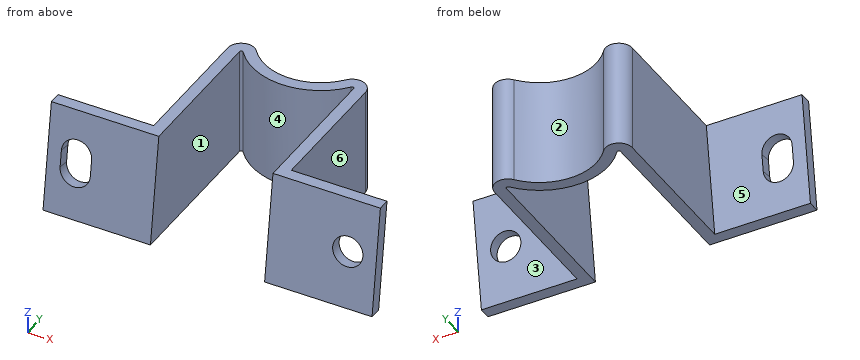
from build123d import *

# Parameters (mm, degrees)
EXTRUDE_1_DEPTH     = 16
CUT_EXTRUDE_1_DEPTH = 50
EXTRUDE_2_DEPTH     = 28.5
SKETCH_4_R          = 4.5
CUT_EXTRUDE_2_DEPTH = 28.5


with BuildPart() as part:
    # 草图1 → 凸台-拉伸1 (new, symmetric)
    with BuildSketch(Plane.XY):
        with BuildLine():
            Line((-17, -12.990381057), (-17, -66.86388681))
            Line((-17, -66.86388681), (-20.5, -66.86388681))
            Line((-20.5, -66.86388681), (-20.5, -12.990381057))
            ThreePointArc((-20.5, -12.990381057), (-17.809307341, -9.210736327), (-13.357142857, -10.51602276))
            ThreePointArc((-13.357142857, -10.51602276), (0, -17), (13.357142857, -10.51602276))
            ThreePointArc((13.357142857, -10.51602276), (17.809307341, -9.210736327), (20.5, -12.990381057))
            Line((20.5, -12.990381057), (20.5, -66.86388681))
            Line((20.5, -66.86388681), (17, -66.86388681))
            Line((17, -66.86388681), (17, -12.990381057))
            ThreePointArc((17, -12.990381057), (16.663663418, -12.517925466), (16.107142857, -12.68108627))
            ThreePointArc((16.107142857, -12.68108627), (0, -20.5), (-16.107142857, -12.68108627))
            ThreePointArc((-16.107142857, -12.68108627), (-16.663663418, -12.517925466), (-17, -12.990381057))
        make_face()
    extrude(amount=EXTRUDE_1_DEPTH, both=True)

    # 草图2 → 切除-拉伸1 (cut, symmetric)
    with BuildSketch(Plane(origin=(0, 0, 0), x_dir=(0, 0, -1), z_dir=(1, 0, 0))):
        Polygon((16, -60.748653355), (-16, -56.251346645), (-16, -66.86388681), (16, -66.86388681), align=None)
    extrude(amount=CUT_EXTRUDE_1_DEPTH, both=True, mode=Mode.SUBTRACT)

    # 草图3 → 凸台-拉伸2 (add)
    with BuildSketch(Plane.ZY.offset(20.5)):
        Polygon((-16, -60.748653355), (16, -56.251346645), (16, -52.716950141), (-16, -57.214256851), align=None)
    extrude_2 = extrude(amount=EXTRUDE_2_DEPTH)

    # 镜向1: 凸台-拉伸2 across plane
    add(extrude_2.mirror(Plane(origin=(0, 0, 0), x_dir=(0, 0, 1), z_dir=(1, 0, 0))))

    # 草图4 → 切除-拉伸2 (cut)
    with BuildSketch(Plane(origin=(0, -53.900966366, 7.575286804), x_dir=(1, 0, 0), z_dir=(0, 0.9902680687415715, -0.13917310096005808))):
        with Locations(Location((40.5, 7.649733485, 0), (0, 0, 270))):
            Circle(SKETCH_4_R)
        with BuildLine():
            Line((-36, 10.149733485), (-36, 5.149733485))
            ThreePointArc((-36, 5.149733485), (-40.5, 0.649733485), (-45, 5.149733485))
            Line((-45, 5.149733485), (-45, 10.149733485))
            ThreePointArc((-45, 10.149733485), (-40.5, 14.649733485), (-36, 10.149733485))
        make_face()
    extrude(amount=-CUT_EXTRUDE_2_DEPTH, mode=Mode.SUBTRACT)


solid = part.part
Read the model definition and answer for the solid it produces. Units are mm, in the model's axes. Face numbers are marked on the shaded views. A direction names the side the tool comes from. Round coordinates to 2 decimals unless told otherwise and drop trailing zeros. Write each loop counter-clockwise with the first axis right and the second up, starting at its lowest first coordinate (ties: lowest second). Pieces come first, ordered by that corner, then holes.
Q1. Find section A-A on y = -36.5. Determine the outline of the cut face in (x, z), and give its area (3 significant figures).
Values:
outline: (-20.5, -16) - (-17, -16) - (-17, 16) - (-20.5, 16) - close; (17, -16) - (20.5, -16) - (20.5, 16) - (17, 16) - close
area: 224 mm2
Q2. Flat-ended cylindrical pins translate along their axes: P1, Ø8, axis at x = -2.5, z = 6, coming from the +Y side; P2, Ø10, axis at y = -30, z = 11.5, coming from the +X side; P3, Ø16, axis at y = -48.5, z = -6.5, coming from the -X side; P4, Ø5, axis at x = -32.5, z = -2, coming from the -Y side. Find the tip coordinate at first contact, or state that the pin passes through.
Values:
P1: stops at y = -15.71
P2: stops at x = 20.5
P3: stops at x = -49
P4: stops at y = -59.13
Q3. Find section C-C on y = -16. Determine the outline of the cut face in (x, z), and give its area (3 significant figures).
Values:
outline: (-20.5, -16) - (-17, -16) - (-17, 16) - (-20.5, 16) - close; (-12.82, -16) - (-5.74, -16) - (-5.74, 16) - (-12.82, 16) - close; (5.74, -16) - (12.82, -16) - (12.82, 16) - (5.74, 16) - close; (17, -16) - (20.5, -16) - (20.5, 16) - (17, 16) - close
area: 677 mm2
Q4. The mould has two halves that part along X. Classify the marked faces 4, 5 and 6: released by +X, released by -X, zero draft, split by the parting line, or undercut.
Values:
face 4: undercut
face 5: zero draft
face 6: released by +X
Q5. Find section D-D on z = -11.5. Determine the outline of the cut face in (x, y), and give its area (3 significant figures).
Values:
outline: (-49, -60.12) - (-17, -60.12) - (-17, -12.99) arc R0.5 cw to (-16.11, -12.68) arc R20.5 ccw to (16.11, -12.68) arc R0.5 cw to (17, -12.99) - (17, -60.12) - (49, -60.12) - (49, -56.58) - (20.5, -56.58) - (20.5, -12.99) arc R4 ccw to (13.36, -10.52) arc R17 cw to (-13.36, -10.52) arc R4 ccw to (-20.5, -12.99) - (-20.5, -56.58) - (-49, -56.58) - close
area: 689 mm2
Q6. A tool of negligible diameter and unlimited length cuts with its end or side. For the marked faces 1, 2 and 3, from which of +Z, -Z, +X, -X, +Y, -Y can it reach the whole face along a straight path? Write none if from no direction.
Values:
face 1: +Z, -Z, -Y
face 2: +Z, -Z, +Y
face 3: -Z, +X, +Y
Q7. Find section B-B on x = -37.5. Determine the outline of the cut face in (y, z), and give its area (3 significant figures).
Values:
outline: (-60.75, -16) - (-57.21, -16) - (-55.78, -5.8) - (-59.25, -5.31) - close; (-57.62, 6.28) - (-54.15, 5.8) - (-52.72, 16) - (-56.25, 16) - close
area: 72.1 mm2
Q8. Straight lines are drawn through the part: line 1 (X direction, y = -31, z = -12); line 2 (X direction, y = -54.5, z = 9.5); line 3 (Y direction, x = 11, z = 9.5). For each, find the intervals that lie inside material, in ascending order.
Values:
line 1: x = -20.5 to -17, 17 to 20.5
line 2: x = -49 to -17, 17 to 49
line 3: y = -17.3 to -12.96
